Geometry check sheet. Reference: the model listing, model coordinates, mm. Coordinates: 2 decimals unless noted, no trailing zeros. Loops run counter-clockwise (first coordinate to the right, second up) from the corner with the lowest first, then second, coordinate; pieces in that order, holes last. Notation, with made-up numbers: (60, 5.25) - (98, 5.25) arc R20 cw to (98, 41.25) - close; hole circle Ø7 at (57.25, 53). An arc over 180 degrees is marked (long way). Write each question's results on one line, items separated by ' | '. Start each with the question number.
(1) Material ranges on probe 1 along X at (y, z) = (1.25, 3.5); probe 2 along X at (y, z) = (2.75, -3.5); probe 3 along Y at (x, z) = (-678, 1), recorded low to high.
(2) Sectioned sample at A-A (x = -121). Enter the section's corners in (y, z).
(3) Go/stop test with flat-tipped pins: pin 1 Ø2 at (y, z) = (-9, -2) entering from -X; pin 2 Ø8 at (x, y) = (-820.5, -5.5) entering from +Z; pin 3 Ø6.5 at (x, z) = (-1282.5, -2.5) entering from +Y (3 decimals). Record where each tip stops, or that it passes through.
from build123d import *

# Parameters (mm, degrees)
EXTRUSION1_DEPTH      = 0.635
EXTRUSION1_DEPTH_BACK = 0.635
SKETCH1_R             = 6.35
EXTRUSION2_DEPTH      = 19.05
EXTRUSION2_DEPTH_BACK = 19.05
SKETCH2_R             = 6.35
SKETCH3_R             = 6.35
EXTRUSION3_DEPTH      = 13.97
SKETCH4_R             = 6.35
EXTRUSION4_DEPTH      = 3.81
SKETCH5_R             = 8.3312
EXTRUSION5_DEPTH      = 1271.27
SKETCH6_R             = 6.35
EXTRUSION6_DEPTH      = 1.27
SKETCH7_R             = 6.35
EXTRUSION7_DEPTH      = 20.32
FILLET1_R             = 7.62


with BuildPart() as part:
    # Sketch1 → Extrusion1 (new, two sides: drawn at the far end of the back side and taken through both)
    with BuildSketch(Plane(origin=(0, 0, 0), x_dir=(-1, 0, 0), z_dir=(0, 1, 0)).offset(-EXTRUSION1_DEPTH_BACK)):
        Polygon((-22.104096049, 6.444983804), (-22.104096049, -6.444983804), (0, -8.3312), (0, 8.3312), align=None)
        with Locations(Location((-9.144, 0, 0), (0, 0, 90))):
            Circle(SKETCH1_R, mode=Mode.SUBTRACT)
    extrude(amount=EXTRUSION1_DEPTH + EXTRUSION1_DEPTH_BACK)

    # Sketch2 → Extrusion2 (add, two sides: drawn at the far end of the back side and taken through both)
    with BuildSketch(Plane.XZ.offset(0.635).offset(-EXTRUSION2_DEPTH_BACK)):
        with Locations(Location((9.144, 0, 0), (0, 0, 270))):
            Circle(SKETCH2_R)
    extrude(amount=EXTRUSION2_DEPTH + EXTRUSION2_DEPTH_BACK)

    # Sketch3 → Extrusion3 (cut)
    with BuildSketch(Plane(origin=(0, 18.415, 0), x_dir=(-1, 0, 0), z_dir=(0, 1, 0))):
        with Locations(Location((-9.144, 0, 0), (0, 0, 270))):
            Circle(SKETCH3_R)
    extrude(amount=-EXTRUSION3_DEPTH, mode=Mode.SUBTRACT)

    # Sketch5 → Extrusion5 (add)
    with BuildSketch(Plane.ZY):
        Circle(SKETCH5_R)
    extrude(amount=EXTRUSION5_DEPTH)

    # Sketch6 → Extrusion6 (add)
    with BuildSketch(Plane.XZ.offset(-0.635)):
        Polygon((-1293.4696, 0), (-1293.4696, -6.477), (-1271.27, -8.3312), (-1271.27, 8.3312), (-1293.4696, 6.477), align=None)
        with Locations(Location((-1280.5156, 0, 0), (0, 0, 90))):
            Circle(SKETCH6_R, mode=Mode.SUBTRACT)
    extrude(amount=EXTRUSION6_DEPTH)



with BuildPart() as body_2:
    # Sketch4 → Extrusion4 (new body)
    with BuildSketch(Plane(origin=(0, 4.445, 0), x_dir=(-1, 0, 0), z_dir=(0, 1, 0))):
        with Locations(Location((1280.5156, 0, 0), (0, 0, 90))):
            Circle(SKETCH4_R)
    extrude(amount=-EXTRUSION4_DEPTH)


with BuildPart() as part_1:
    add(part.part)

    add(body_2.part)  # Extrusion7 merges body 2
    # Sketch7 → Extrusion7 (add)
    with BuildSketch(Plane.XZ.offset(-0.635)):
        with Locations(Location((-1280.5156, 0, 0), (0, 0, 270))):
            Circle(SKETCH7_R)
    extrude(amount=EXTRUSION7_DEPTH)

    # Fillet1
    # the kernel refuses this fillet: 7.62 mm, written as the material it takes off along each edge
    with BuildSketch(Plane(origin=(-1271.27, 0, 0), x_dir=(0, -0.9999950652018581, 0.003141587485873656), z_dir=(0, -0.003141587485873656, -0.9999950652018581))) as fillet1_piece_1_section:
        with BuildLine():
            CenterArc((8.3312 - FILLET1_R, -FILLET1_R), FILLET1_R, 0, 90)
            Line((8.3312 - FILLET1_R, 0), (8.3312, 0))
            Line((8.3312, 0), (8.3312, -FILLET1_R))
        make_face()
    fillet1_piece_1 = revolve(axis=Axis((-1271.27, 0, 0), (-1, 0, 0)), revolution_arc=359.64, mode=Mode.PRIVATE)
    fillet1_piece_1 = split(fillet1_piece_1, bisect_by=Plane(origin=(-1269.374883086, -0.635, 4.28224122), z_dir=(0, -1, 0)), keep=Keep.TOP, mode=Mode.PRIVATE)
    add(fillet1_piece_1, mode=Mode.SUBTRACT)
    with BuildSketch(Plane(origin=(-1271.27, 0, 0), x_dir=(0, -0.9999950652018581, 0.003141587485873656), z_dir=(0, -0.003141587485873656, -0.9999950652018581))) as fillet1_piece_2_section:
        with BuildLine():
            CenterArc((8.3312 - FILLET1_R, -FILLET1_R), FILLET1_R, 0, 90)
            Line((8.3312 - FILLET1_R, 0), (8.3312, 0))
            Line((8.3312, 0), (8.3312, -FILLET1_R))
        make_face()
    fillet1_piece_2 = revolve(axis=Axis((-1271.27, 0, 0), (-1, 0, 0)), revolution_arc=359.64, mode=Mode.PRIVATE)
    fillet1_piece_2 = split(fillet1_piece_2, bisect_by=Plane(origin=(-1269.082318262, 0.635, 0), z_dir=(0, 1, 0)), keep=Keep.TOP, mode=Mode.PRIVATE)
    add(fillet1_piece_2, mode=Mode.SUBTRACT)
    with BuildSketch(Plane(origin=(0, 0, 0), x_dir=(0, -0.9999950652018581, 0.003141587485874322), z_dir=(0, -0.003141587485874322, -0.9999950652018581))) as fillet1_piece_3_section:
        with BuildLine():
            CenterArc((8.3312 - FILLET1_R, FILLET1_R), FILLET1_R, 270, 90)
            Line((8.3312, FILLET1_R), (8.3312, 0))
            Line((8.3312, 0), (8.3312 - FILLET1_R, 0))
        make_face()
    fillet1_piece_3 = revolve(axis=Axis((0, 0, 0), (-1, 0, 0)), revolution_arc=359.64, mode=Mode.PRIVATE)
    fillet1_piece_3 = split(fillet1_piece_3, bisect_by=Plane(origin=(-1.895117191, -0.635, 4.282241186), z_dir=(0, -1, 0)), keep=Keep.TOP, mode=Mode.PRIVATE)
    add(fillet1_piece_3, mode=Mode.SUBTRACT)
    with BuildSketch(Plane(origin=(0, 0, 0), x_dir=(0, -0.9999950652018581, 0.003141587485874322), z_dir=(0, -0.003141587485874322, -0.9999950652018581))) as fillet1_piece_4_section:
        with BuildLine():
            CenterArc((8.3312 - FILLET1_R, FILLET1_R), FILLET1_R, 270, 90)
            Line((8.3312, FILLET1_R), (8.3312, 0))
            Line((8.3312, 0), (8.3312 - FILLET1_R, 0))
        make_face()
    fillet1_piece_4 = revolve(axis=Axis((0, 0, 0), (-1, 0, 0)), revolution_arc=359.64, mode=Mode.PRIVATE)
    fillet1_piece_4 = split(fillet1_piece_4, bisect_by=Plane(origin=(-2.187681733, 0.635, 0), z_dir=(0, 1, 0)), keep=Keep.TOP, mode=Mode.PRIVATE)
    add(fillet1_piece_4, mode=Mode.SUBTRACT)
    with BuildSketch(Plane(origin=(0, 0, 0), x_dir=(0, 0.9999950652018581, -0.00314158748588508), z_dir=(0, 0.00314158748588508, 0.9999950652018581))) as fillet1_piece_5_section:
        with BuildLine():
            CenterArc((8.3312 - FILLET1_R, FILLET1_R), FILLET1_R, 270, 90)
            Line((8.3312, FILLET1_R), (8.3312, 0))
            Line((8.3312, 0), (8.3312 - FILLET1_R, 0))
        make_face()
    fillet1_piece_5 = revolve(axis=Axis((0, 0, 0), (-1, 0, 0)), revolution_arc=359.64, mode=Mode.PRIVATE)
    fillet1_piece_5 = split(fillet1_piece_5, bisect_by=Plane(origin=(-1.895117191, 0.635, -4.282241186), z_dir=(0, 1, 0)), keep=Keep.TOP, mode=Mode.PRIVATE)
    add(fillet1_piece_5, mode=Mode.SUBTRACT)
    with BuildSketch(Plane(origin=(0, 0, 0), x_dir=(0, 0.9999950652018581, -0.00314158748588508), z_dir=(0, 0.00314158748588508, 0.9999950652018581))) as fillet1_piece_6_section:
        with BuildLine():
            CenterArc((8.3312 - FILLET1_R, FILLET1_R), FILLET1_R, 270, 90)
            Line((8.3312, FILLET1_R), (8.3312, 0))
            Line((8.3312, 0), (8.3312 - FILLET1_R, 0))
        make_face()
    fillet1_piece_6 = revolve(axis=Axis((0, 0, 0), (-1, 0, 0)), revolution_arc=359.64, mode=Mode.PRIVATE)
    fillet1_piece_6 = split(fillet1_piece_6, bisect_by=Plane(origin=(-2.187681733, -0.635, 0), z_dir=(0, -1, 0)), keep=Keep.TOP, mode=Mode.PRIVATE)
    add(fillet1_piece_6, mode=Mode.SUBTRACT)
    with BuildSketch(Plane(origin=(-1271.27, 0, 0), x_dir=(0, 0.9999950652018581, -0.003141587485884858), z_dir=(0, 0.003141587485884858, 0.9999950652018581))) as fillet1_piece_7_section:
        with BuildLine():
            CenterArc((8.3312 - FILLET1_R, -FILLET1_R), FILLET1_R, 0, 90)
            Line((8.3312 - FILLET1_R, 0), (8.3312, 0))
            Line((8.3312, 0), (8.3312, -FILLET1_R))
        make_face()
    fillet1_piece_7 = revolve(axis=Axis((-1271.27, 0, 0), (-1, 0, 0)), revolution_arc=359.64, mode=Mode.PRIVATE)
    fillet1_piece_7 = split(fillet1_piece_7, bisect_by=Plane(origin=(-1269.374883188, 0.635, -4.282241233), z_dir=(0, 1, 0)), keep=Keep.TOP, mode=Mode.PRIVATE)
    add(fillet1_piece_7, mode=Mode.SUBTRACT)
    with BuildSketch(Plane(origin=(-1271.27, 0, 0), x_dir=(0, 0.9999950652018581, -0.003141587485884858), z_dir=(0, 0.003141587485884858, 0.9999950652018581))) as fillet1_piece_8_section:
        with BuildLine():
            CenterArc((8.3312 - FILLET1_R, -FILLET1_R), FILLET1_R, 0, 90)
            Line((8.3312 - FILLET1_R, 0), (8.3312, 0))
            Line((8.3312, 0), (8.3312, -FILLET1_R))
        make_face()
    fillet1_piece_8 = revolve(axis=Axis((-1271.27, 0, 0), (-1, 0, 0)), revolution_arc=359.64, mode=Mode.PRIVATE)
    fillet1_piece_8 = split(fillet1_piece_8, bisect_by=Plane(origin=(-1269.082318263, -0.635, 0), z_dir=(0, -1, 0)), keep=Keep.TOP, mode=Mode.PRIVATE)
    add(fillet1_piece_8, mode=Mode.SUBTRACT)


solid = part_1.part
Outcome:
1) probe 1: x = -1285.81 to -1275.22, -1270.65 to -0.62, 3.85 to 14.44 | probe 2: x = -1285.81 to -1275.22, -1270.29 to -0.98, 3.85 to 14.44 | probe 3: y = -8.27 to 8.27
2) outline: circle Ø16.66 at (0, 0)
3) pin 1: stops at x = -1286.79 | pin 2: stops at z = 8.2 | pin 3: stops at y = 4.445
